Geometry check sheet. Reference: the model listing, model coordinates, mm. Face numbers are marked on the shaded views. A direction names the side the tool comes from. Coordinates: 2 decimals unless noted, no trailing zeros. Order: outer loops, then holes, each group sorted by start corner. A loop starts at its lowest first (then second) coordinate and runs counter-clockwise, first axis right, second up. Notation, with made-up numbers: M -17.75,-0.75 L 6.25,-0.75 A19 ccw 6.25,32.25 Z; hole C -37,9.25 d7. An arc over 180 degrees is marked long. Use CSV: the item, a comma, the result in double quotes. Start each with the question number.
Autodesk Inventor part; units mm, degrees
ref_plane "YZ Plane" through (0, 0, 0) normal (1, 0, 0) x (0, 1, 0)
ref_plane "XZ Plane" through (0, 0, 0) normal (0, 1, 0) x (-1, 0, 0)
ref_plane "XY Plane" through (0, 0, 0) normal (0, 0, 1) x (1, 0, 0)
sketch "Esboço1" plane through (0, 0, 0) normal (0, 0, 1) x (1, 0, 0)
  line L0 (0, 0) -> (70, 0)
  line L1 (70, 0) -> (70, 35)
  line L2 (70, 35) -> (0, 35)
  line L3 (0, 35) -> (0, 0)
  dimension "d0" = 70
  dimension "d1" = 35
extrude "Extrusão1" add sketch "Esboço1" along normal blind 10
fillet "Arredondamento1" radius 3 4 edges at (70, 35, 5) (70, 0, 5) (0, 35, 5) (0, 0, 5)
fillet "Arredondamento2" radius 3 8 edges at (0.8787, 34.1213, 0) (0, 17.5, 0) (0.8787, 0.8787, 0) (35, 0, 0) (69.1213, 0.8787, 0) (70, 17.5, 0) (69.1213, 34.1213, 0) (35, 35, 0)
shell "Casca1" thickness 1 removed faces 1 at (45.6667, 11.6667, 10)
sketch "Esboço2" plane through (0, 0, 0) normal (0, 0, -1) x (-1, 0, 0)
  circle A0 centre (-7, 7) radius 1.5
  line L0 (-3, 3) -> (-67, 3)
  line L1 (-3, 32) -> (-3, 3)
  point P0 (0, 0)
  dimension "d7" = 3
  dimension "d8" = 4
  dimension "d9" = 4
extrude "Extrusão2" cut sketch "Esboço2" against normal through all
pattern_linear "Padrão retangular1" count 6 spacing 11 along (1, 0, 0) count 4 spacing 6 along (0, 1, 0) of "Extrusão2"
properties part number "Peça2-Rubia"
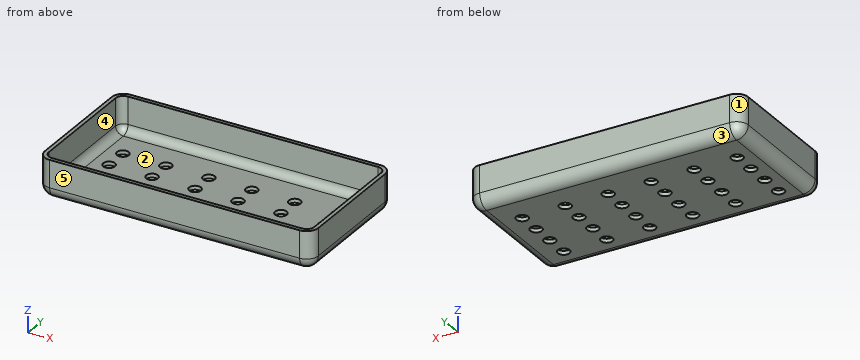
1) Section check D-D on x = 14.5. Record the boundary of the cut face in (y, z), then the cut area to 3 significant figures.
2) Gauge pin test, flat ends, axial feed: P1, Ø5, axis at x = 51, y = 13, coming from the +Z side; P2, Ø2.5, axis at x = 18, y = 19, coming from the +Z side; P3, Ø1.5, axis at x = 56, z = 1.5, coming from the -Y side. Record the tip position at first contact, or that the pin passes through.
3) Draft check along X on the marked faces 1, 2 and 3. Enter one of: +X half, -X half, draft (parallel to the pull), parting line (faces both ways), or undercut.
4) Section check B-B on z = 4.75. Record the boundary of the cut face in (x, y).
5) Set-up check for the marked faces 4 and 5: record each of +Z, -Z, +X, -X, +Y, -Y from which the full face is reachable in a straight line by a thin tool's end or side.
6) Section check A-A on x = 29. Record the boundary of the cut face in (y, z).
7) Material ranges on line 1 along X through (y, z) = (15, 7.5); line 2 along Y through (x, z) = (23.5, 3.5); line 3 along Y through (x, z) = (7, 0.45), recorded low to high.
8) Section check C-C on y = 4. Record the boundary of the cut face in (x, z).
Results are:
1,outline,"M 0,3 A3 ccw 3,0 L 32,0 A3 ccw 35,3 L 35,10 L 34,10 L 34,3 A2 cw 32,1 L 3,1 A2 cw 1,3 L 1,10 L 0,10 Z"
1,area,"50.9 mm²"
2,P1,"stops at z = 1"
2,P2,"passes through"
2,P3,"stops at y = 0.1"
3,face 1,"-X half"
3,face 2,"undercut"
3,face 3,"draft"
4,outline,"M 0,3 A3 ccw 3,0 L 67,0 A3 ccw 70,3 L 70,32 A3 ccw 67,35 L 3,35 A3 ccw 0,32 Z; hole M 1,3 A2 ccw 3,1 L 67,1 A2 ccw 69,3 L 69,32 A2 ccw 67,34 L 3,34 A2 ccw 1,32 Z"
5,face 4,"+Z"
5,face 5,"+Z, -Z, +X, -X, -Y"
6,outline,"M 0,3 A3 ccw 3,0 L 5.5,0 L 5.5,1 L 3,1 A2 cw 1,3 L 1,10 L 0,10 Z; M 8.5,0 L 11.5,0 L 11.5,1 L 8.5,1 Z; M 14.5,0 L 17.5,0 L 17.5,1 L 14.5,1 Z; M 20.5,0 L 23.5,0 L 23.5,1 L 20.5,1 Z; M 26.5,0 L 32,0 A3 ccw 35,3 L 35,10 L 34,10 L 34,3 A2 cw 32,1 L 26.5,1 Z"
7,line 1,"x = 0 to 1, 69 to 70"
7,line 2,"y = 0 to 1, 34 to 35"
7,line 3,"y = 1.42 to 5.5, 8.5 to 11.5, 14.5 to 17.5, 20.5 to 23.5, 26.5 to 33.58"
8,outline,"M 0,3 A3 ccw 3,0 L 67,0 A3 ccw 70,3 L 70,10 L 69,10 L 69,3 A2 cw 67,1 L 3,1 A2 cw 1,3 L 1,10 L 0,10 Z"
